Study the drawing (mm; zero at the part's minimum x, y, z) and answer. A direction names the side the tool comes from. Give positions to 0.01 mm unless a question says otherwise; leave off trailing zeros. Loops run counter-clockwise (first coordinate to the right, second up) from the corner with the lowest first, then second, coordinate; pieces in that order, holes last. Notation, with made-up numbers: (21.5, 73) - (49.5, 73) arc R32 ccw to (49.5, 99) - close; hole circle Ø11 at (59.25, 11.25). An arc over 180 degrees is marked (long way). Answer in a Markdown table with one row per item. Add a question column.
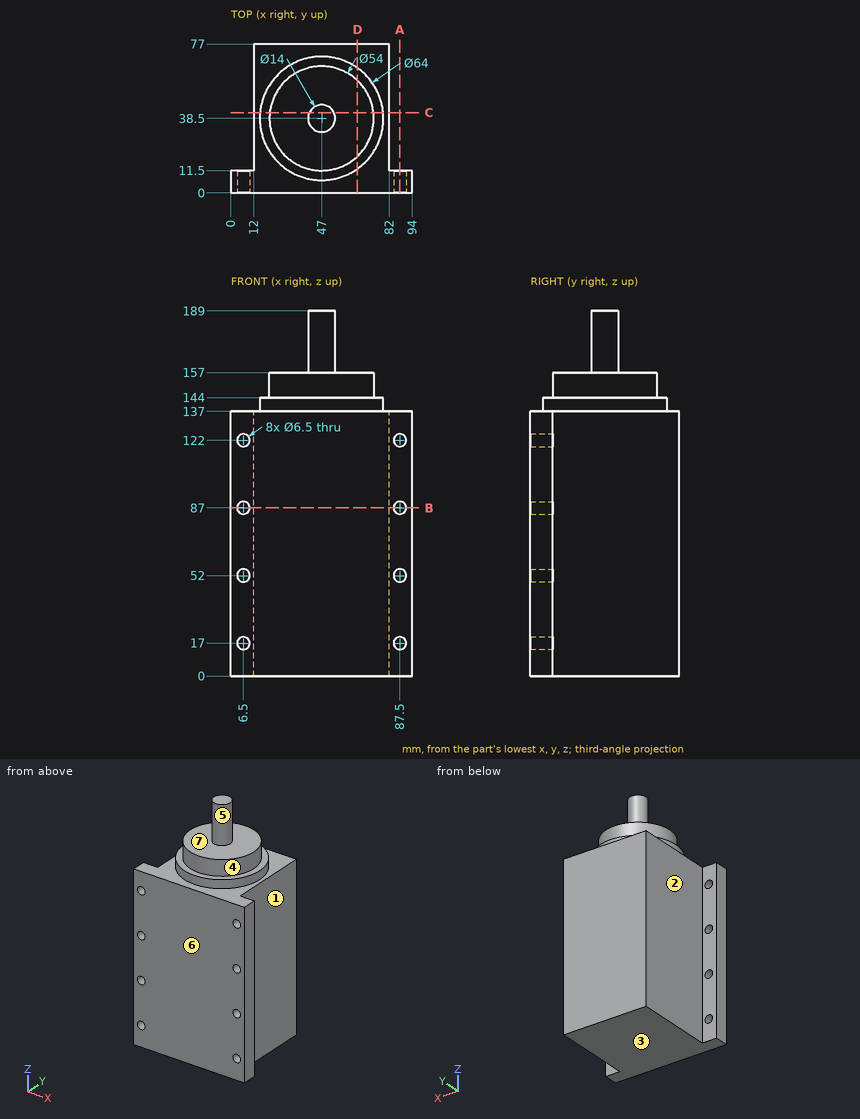
(1) A cutting plane is placed at B-B on z = 87. Determine the outline of the cut face in (x, y).
(2) Find the intervals of material crossed by line 1 along Z through (x, y) = (87, 7); line 2 along X through (y, z) = (3, 52); line 3 along Z through (x, y) = (31, 66.5), in increasing order. Write a range as [from, to].
(3) A cutting plane is placed at C-C on y = 41.5. Determine the outline of the cut face in (x, z), plus the area to 3 significant figures.
(4) A cutting plane is placed at D-D on x = 65.5. Determine the outline of the cut face in (y, z).
(5) Given pin 1 Ø5 at (x, z) = (87.5, 17) entering from +Y; pin 2 Ø8.5 at (x, z) = (87.5, 52) entering from +Y; pin 3 Ø2 at (y, z) = (48, 142.5) entering from -X; pin 4 Ø10 at (y, z) = (43, 141.5) entering from +X, each flat-ended and moving along its own axis, determine where each tip first touches the part or whether it passes through.
(6) A cutting plane is placed at A-A on x = 87.5. Determine the outline of the cut face in (y, z).
(7) A tool of negligible diameter and unlimited length cuts with its end or side. For the marked faces 1, 2, 3 and 4, from which of +Z, -Z, +X, -X, +Y, -Y can it reach the whole face along a straight path? Write none if from no direction.
(8) The mould has two halves that part along Y. Classify the marked faces 5, 6 and 7: pulls with the +Y half, pulls with the -Y half, needs draft (parallel to the pull), parting line crosses it, or undercut.
Evaluation:
| question | item | result |
|---|---|---|
| 1 | outline | (0, 0) - (3.25, 0) - (3.25, 11.5) - (0, 11.5) - close; (9.75, 0) - (84.25, 0) - (84.25, 11.5) - (82, 11.5) - (82, 77) - (12, 77) - (12, 11.5) - (9.75, 11.5) - close; (90.75, 0) - (94, 0) - (94, 11.5) - (90.75, 11.5) - close |
| 2 | line 1 | z = [0, 13.79], [20.21, 48.79], [55.21, 83.79], [90.21, 118.79], [125.21, 137] |
| 2 | line 2 | x = [0, 3.25], [9.75, 84.25], [90.75, 94] |
| 2 | line 3 | z = [0, 137] |
| 3 | outline | (12, 0) - (82, 0) - (82, 137) - (78.86, 137) - (78.86, 144) - (73.83, 144) - (73.83, 157) - (53.32, 157) - (53.32, 189) - (40.68, 189) - (40.68, 157) - (20.17, 157) - (20.17, 144) - (15.14, 144) - (15.14, 137) - (12, 137) - close |
| 3 | area | 11,100 mm² |
| 4 | outline | (0, 0) - (77, 0) - (77, 137) - (64.61, 137) - (64.61, 144) - (58.17, 144) - (58.17, 157) - (18.83, 157) - (18.83, 144) - (12.39, 144) - (12.39, 137) - (0, 137) - close |
| 5 | pin 1 | passes through |
| 5 | pin 2 | stops at y = 11.5 |
| 5 | pin 3 | stops at x = 16.15 |
| 5 | pin 4 | stops at x = 82 |
| 6 | outline | (0, 0) - (11.5, 0) - (11.5, 13.75) - (0, 13.75) - close; (0, 20.25) - (11.5, 20.25) - (11.5, 48.75) - (0, 48.75) - close; (0, 55.25) - (11.5, 55.25) - (11.5, 83.75) - (0, 83.75) - close; (0, 90.25) - (11.5, 90.25) - (11.5, 118.75) - (0, 118.75) - close; (0, 125.25) - (11.5, 125.25) - (11.5, 137) - (0, 137) - close |
| 7 | face 1 | +Z, -Z, +X, +Y |
| 7 | face 2 | +Z, -Z, -X, +Y |
| 7 | face 3 | -Z, +X, -X, +Y, -Y |
| 7 | face 4 | +Z |
| 8 | face 5 | parting line crosses it |
| 8 | face 6 | pulls with the -Y half |
| 8 | face 7 | needs draft |
